Source: CAD feature listing. Evaluate the final solid. Frame: model axes, mm. A direction names the side the tool comes from. Coordinates: 2 decimals unless noted, no trailing zeros. Write each loop counter-clockwise with the first axis right and the second up, starting at its lowest first coordinate (ties: lowest second). Pieces come first, ordered by that corner, then holes. Notation, with made-up numbers: M -14,-31 L 34,-31 A18 ccw 34,-12 Z; hole C 86.25,-38 d11. An arc over 180 degrees is marked long. Answer as CSV lines item,"result". Start each with the question number.
1. Reachability of faces 3 (the face through (17.22, -1.48, -7.85)), 4 (the face through (0, -17, -1.75)) from +Z, -Z, +X, -X, +Y, -Y: full face, straight path, thin tool, end or side. Return the list, or none.
2. Section B-B on x = 0. Return the cut outline in (y, z).
3. Section D-D on z = -28. Return the cut outline in (x, y).
4. Section C-C on z = -18. Return the cut outline in (x, y).
5. Section A-A on y = -20.5. Return the cut outline in (x, z).
6. Contact query for flat-ended pins moving along their axis: pin 1 Ø6 at (x, z) = (-20, -12.5) entering from -Y; pin 2 Ø2 at (x, y) = (23.5, -10.5) entering from -Z; pin 3 Ø1.3 at (x, y) = (-1, -20) entering from -Z. Output: stop coordinate, or through.
7. Mould query, pull axis X, two halves, no side actions, for faces 1 (the face through (0, -3, 0)), 2 (the face through (0, 0, 0)). Classes: pulls with the +X half, pulls with the -X half, needs draft (parallel to the pull), parting line crosses it, or undercut.
8. Line query: probe 1 along Y at (x, z) = (-20.5, -5); probe 2 along Y at (x, z) = (11.5, 20.5); probe 3 along Z at (x, y) = (-1, -25). Output: solid intervals per line, ascending. Write a range as [from, to].
```python
from build123d import *

# Parameters (mm, degrees)
F0_R     = 8.75
F1_DEPTH = 3
F0_R_2   = 35
F2_DEPTH = 28
F3_R     = 5
F4_DEPTH = 28.5


with BuildPart() as f1:
    # F0 (on Front) → F1 (new body)
    with BuildSketch(Plane.XZ):
        with BuildLine():
            Line((11.2055757109, 10.7121584512), (14.409271678, 17.2807085997))
            ThreePointArc((14.409271678, 17.2807085997), (13.2255061098, 18.2026368458), (11.9829277906, 19.043619445))
            Line((11.9829277906, 19.043619445), (6.7263225873, 13.9673748066))
            ThreePointArc((6.7263225873, 13.9673748066), (0.0005839076, 11.2499999919), (-6.7251547721, 13.9673748066))
            Line((-6.7251547721, 13.9673748066), (-11.9822206949, 19.0440643566))
            ThreePointArc((-11.9822206949, 19.0440643566), (-13.2248302388, 18.2031278948), (-14.4086300373, 17.2812436025))
            Line((-14.4086300373, 17.2812436025), (-11.2052148362, 10.7132691094))
            ThreePointArc((-11.2052148362, 10.7132691094), (-10.6992053632, 3.4769965133), (-15.3619499397, -2.0798460871))
            Line((-15.3619499397, -2.0798460871), (-21.8146913282, -5.5108295434))
            ThreePointArc((-21.8146913282, -5.5108295434), (-21.3989006928, -6.9524851052), (-20.887950885, -8.3632235308))
            Line((-20.887950885, -8.3632235308), (-13.6515262074, -7.3462103663))
            ThreePointArc((-13.6515262074, -7.3462103663), (-6.6130564747, -9.1010979679), (-2.7690524241, -15.2527903798))
            Line((-2.7690524241, -15.2527903798), (-1.5, -22.4499443206))
            ThreePointArc((-1.5, -22.4499443206), (-0.0004177112, -22.4999999961), (1.4991664351, -22.45))
            Line((1.4991664351, -22.45), (2.7681076417, -15.2534768043))
            ThreePointArc((2.7681076417, -15.2534768043), (6.6121116923, -9.1017843924), (13.650581425, -7.3468967909))
            Line((13.650581425, -7.3468967909), (20.887640345, -8.3639990923))
            ThreePointArc((20.887640345, -8.3639990923), (21.3986425331, -6.9532796392), (21.8144866967, -5.5116395166))
            Line((21.8144866967, -5.5116395166), (15.3623108145, -2.0809567454))
            ThreePointArc((15.3623108145, -2.0809567454), (10.6995662379, 3.4758858551), (11.2055757109, 10.7121584512))
        make_face()
        Circle(F0_R, mode=Mode.SUBTRACT)
        Circle(F0_R)
        Polygon((-3.4579752893, 1.1235642806), (0, 3.635930389), (3.4579752893, 1.1235642806), (2.137146261, -2.9415294751), (-2.137146261, -2.9415294751), align=None, mode=Mode.SUBTRACT)
        Polygon((3.4579752893, 1.1235642806), (0, 3.635930389), (-3.4579752893, 1.1235642806), (-2.137146261, -2.9415294751), (2.137146261, -2.9415294751), align=None)
    extrude(amount=F1_DEPTH)

    # F0 (on Front) → F2 (join)
    with BuildSketch(Plane.XZ):
        Circle(F0_R_2)
        with BuildLine():
            ThreePointArc((14.409271678, 17.2807085997), (20.3771761139, 9.540476593), (22.5, 0))
            ThreePointArc((22.5, 0), (22.3279639765, -2.7770532337), (21.8144866967, -5.5116395166))
            ThreePointArc((21.8144866967, -5.5116395166), (21.3986425331, -6.9532796392), (20.887640345, -8.3639990923))
            ThreePointArc((20.887640345, -8.3639990923), (13.2248302388, -18.2031278948), (1.4991664351, -22.45))
            ThreePointArc((1.4991664351, -22.45), (-0.0004177112, -22.4999999961), (-1.5, -22.4499443206))
            ThreePointArc((-1.5, -22.4499443206), (-13.2255061098, -18.2026368458), (-20.887950885, -8.3632235308))
            ThreePointArc((-20.887950885, -8.3632235308), (-21.3989006928, -6.9524851052), (-21.8146913282, -5.5108295434))
            ThreePointArc((-21.8146913282, -5.5108295434), (-21.3986425331, 6.9532796392), (-14.4086300373, 17.2812436025))
            ThreePointArc((-14.4086300373, 17.2812436025), (-13.2248302388, 18.2031278948), (-11.9822206949, 19.0440643566))
            ThreePointArc((-11.9822206949, 19.0440643566), (0.0004177112, 22.4999999961), (11.9829277906, 19.043619445))
            ThreePointArc((11.9829277906, 19.043619445), (13.2255061098, 18.2026368458), (14.409271678, 17.2807085997))
        make_face(mode=Mode.SUBTRACT)
    extrude(amount=F2_DEPTH)

    # F3 (on face) → F4 (join)
    with BuildSketch(Plane.XZ.offset(3)):
        Circle(F3_R)
        with BuildLine():
            ThreePointArc((2.1213203436, 1.75), (2.5880621075, 0.9297497123), (2.75, 0))
            ThreePointArc((2.75, 0), (2.5880621075, -0.9297497123), (2.1213203436, -1.75))
            ThreePointArc((2.1213203436, -1.75), (0, -2.75), (-2.1213203436, -1.75))
            ThreePointArc((-2.1213203436, -1.75), (-2.75, 0), (-2.1213203436, 1.75))
            ThreePointArc((-2.1213203436, 1.75), (0, 2.75), (2.1213203436, 1.75))
        make_face(mode=Mode.SUBTRACT)
        with BuildLine():
            Line((-2.1213203436, 1.75), (2.1213203436, 1.75))
            ThreePointArc((2.1213203436, 1.75), (0, 2.75), (-2.1213203436, 1.75))
        make_face()
        with BuildLine():
            ThreePointArc((-2.1213203436, -1.75), (0, -2.75), (2.1213203436, -1.75))
            Line((2.1213203436, -1.75), (-2.1213203436, -1.75))
        make_face()
    extrude(amount=F4_DEPTH)


solid = f1.part
```
Values:
1,face 3,"+Y, -Y"
1,face 4,"-Y"
2,outline,"M -31.5,-5 L -3,-5 L -3,-22.5 L -28,-22.5 L -28,-35 L 0,-35 L 0,11.25 L -3,11.25 L -3,5 L -31.5,5 L -31.5,1.75 L -3,1.75 L -3,-1.75 L -31.5,-1.75 Z; M -28,22.5 L 0,22.5 L 0,35 L -28,35 Z"
3,outline,"M -21,-28 L 21,-28 L 21,0 L -21,0 Z"
4,outline,"M -30.02,-28 L -13.5,-28 L -13.5,0 L -30.02,0 Z; M -2.28,-3 L 2.28,-3 L 2.28,0 L -2.28,0 Z; M 13.5,-28 L 30.02,-28 L 30.02,0 L 13.5,0 Z"
5,outline,"C 0,0 d70; C 0,0 d10; hole C 0,0 d45; hole M -2.12,-1.75 L 2.12,-1.75 A2.75 ccw 2.12,1.75 L -2.12,1.75 A2.75 ccw Z"
6,pin 1,"y = -28"
6,pin 2,"z = -26.81"
6,pin 3,"z = -35"
7,face 1,"undercut"
7,face 2,"needs draft"
8,probe 1,"[-3, 0]"
8,probe 2,"[-28, 0]"
8,probe 3,"[-34.99, -22.48], [-4.9, -1.75], [1.75, 4.9], [22.48, 34.99]"
